Build history of the part. All positions in model axes, mm. A direction names the side the tool comes from. Round coordinates to 2 decimals unless told otherwise and drop trailing zeros. Write each loop counter-clockwise with the first axis right and the second up, starting at its lowest first coordinate (ties: lowest second). Pieces come first, ordered by that corner, then holes. Notation, with made-up numbers: M 50.5,72.25 L 89.5,72.25 A26 cw 89.5,100.25 Z; hole C 31,-17.5 d11. An arc over 180 degrees is marked long. Use a Markdown table: item, result.
from build123d import *

# Parameters (mm, degrees)
SKETCH1_R           = 5
BOSS_EXTRUDE1_DEPTH = 30
CUT_EXTRUDE1_DEPTH  = 1


with BuildPart() as part:
    # Sketch1 → Boss-Extrude1 (new body)
    with BuildSketch(Plane(origin=(0, 0, 0), x_dir=(1, 0, 0), z_dir=(0, 1, 0))):
        Circle(SKETCH1_R)
    extrude(amount=BOSS_EXTRUDE1_DEPTH)

    # Sketch2 → Cut-Extrude1 (cut)
    with BuildSketch(Plane(origin=(0, 30, 0), x_dir=(1, 0, 0), z_dir=(0, 1, 0))):
        Polygon((-1.836629209, 1.610053215), (-1.189493792, 1.610053215), (-1.189493792, -1.889946785), (-1.503596356, -1.889946785), (-1.503596356, 1.251078856), (-2.042057895, 1.251078856), align=None)
        with BuildLine():
            add(Edge.make_bspline(
                [(0.111788259, -0.141349029), (0.112116277, -0.085251641), (0.112753457, 0.023718343), (0.119841878, 0.182502986), (0.131617221, 0.331463275), (0.147754593, 0.470606341), (0.167392574, 0.599968105), (0.19360806, 0.719202862), (0.223420863, 0.828862469), (0.257973309, 0.929304517), (0.296961098, 1.02188222), (0.339395358, 1.108307422), (0.386960153, 1.188449354), (0.436937066, 1.263587144), (0.491349137, 1.332490839), (0.548647928, 1.396133502), (0.611069804, 1.453044252), (0.676492812, 1.504890555), (0.745509277, 1.550340026), (0.816151943, 1.590372765), (0.888907049, 1.624572632), (0.963973232, 1.651463068), (1.04067579, 1.673673915), (1.119282856, 1.688862862), (1.19992422, 1.698419771), (1.254355655, 1.699333439), (1.281960535, 1.699796805)],
                knots=[0, 0, 0, 0, 0.000168282, 0.000326891, 0.000476705, 0.00061646, 0.000747059, 0.00086904, 0.000982494, 0.001087814, 0.001187428, 0.001283689, 0.001376399, 0.001466822, 0.001554203, 0.001639568, 0.001723424, 0.001807301, 0.001889751, 0.001971063, 0.002050735, 0.002130583, 0.002210036, 0.002290062, 0.002370508, 0.002453288, 0.002453288, 0.002453288, 0.002453288], degree=3))
            add(Edge.make_bspline(
                [(1.281960535, 1.699796805), (1.309796013, 1.69930899), (1.365152022, 1.698338879), (1.446992397, 1.689014936), (1.526942079, 1.673543813), (1.604660218, 1.651622839), (1.680785204, 1.624427162), (1.754721612, 1.590340045), (1.826928694, 1.550661177), (1.896258981, 1.5040373), (1.963473596, 1.452055024), (2.026921559, 1.393292355), (2.086608645, 1.328342636), (2.143283951, 1.257900772), (2.195339548, 1.180615687), (2.24491298, 1.097831577), (2.289285016, 1.008100712), (2.332019691, 0.912920245), (2.368906678, 0.809656586), (2.402172923, 0.698891825), (2.429051892, 0.579317638), (2.451441164, 0.451561393), (2.46878606, 0.31515391), (2.481418702, 0.170387594), (2.488091787, 0.017167204), (2.489348488, -0.087590645), (2.489993387, -0.141349029)],
                knots=[0, 0, 0, 0, 8.3481e-05, 0.000166017, 0.000246731, 0.000327534, 0.000408041, 0.000488986, 0.000571522, 0.000654944, 0.000739373, 0.000826202, 0.000914021, 0.001003809, 0.001097153, 0.001193347, 0.001293057, 0.001397277, 0.001506176, 0.001621751, 0.001744038, 0.001873599, 0.002010742, 0.002156422, 0.002309427, 0.002470709, 0.002470709, 0.002470709, 0.002470709], degree=3))
            add(Edge.make_bspline(
                [(2.489993387, -0.141349029), (2.489341803, -0.194872936), (2.488072217, -0.299162088), (2.48149351, -0.451693064), (2.468534879, -0.595691107), (2.452324891, -0.731501569), (2.429873928, -0.858559188), (2.402268761, -0.977303637), (2.371618439, -1.088247708), (2.333783644, -1.19048252), (2.292372934, -1.285434243), (2.247317738, -1.374101391), (2.199047912, -1.457267684), (2.146459167, -1.534267431), (2.090405754, -1.605646088), (2.029687965, -1.670143711), (1.96601738, -1.729314382), (1.898604964, -1.78196601), (1.828193413, -1.828050815), (1.756234336, -1.869264665), (1.681450952, -1.90249736), (1.605538, -1.931032401), (1.527409634, -1.952832853), (1.447163243, -1.967906708), (1.365207007, -1.978478557), (1.309805442, -1.979285037), (1.281960535, -1.979690375)],
                knots=[0, 0, 0, 0, 0.000160581, 0.000312886, 0.000457868, 0.000594226, 0.000723097, 0.000844701, 0.000959884, 0.001068125, 0.001171421, 0.001270505, 0.001366343, 0.001459687, 0.001550023, 0.00163832, 0.001725149, 0.001810562, 0.001894568, 0.001977446, 0.00205903, 0.002139777, 0.00222058, 0.002301983, 0.002384599, 0.00246808, 0.00246808, 0.00246808, 0.00246808], degree=3))
            add(Edge.make_bspline(
                [(1.281960535, -1.979690375), (1.254356421, -1.979224019), (1.199926496, -1.978304457), (1.119274071, -1.968790726), (1.040991627, -1.953495223), (0.964692873, -1.932078618), (0.889986358, -1.905863782), (0.817890071, -1.871710099), (0.747602388, -1.83237603), (0.679310832, -1.787580608), (0.614298671, -1.736258925), (0.552200065, -1.679494636), (0.494575046, -1.615871225), (0.440940951, -1.546393302), (0.389966862, -1.47170006), (0.343077489, -1.390771687), (0.299706635, -1.303929076), (0.260063144, -1.210611165), (0.224914481, -1.109456238), (0.193866773, -0.999307059), (0.169352615, -0.879191423), (0.14836966, -0.750074056), (0.131445277, -0.611400125), (0.119890952, -0.463094347), (0.112749637, -0.305249138), (0.112114566, -0.196979364), (0.111788259, -0.141349029)],
                knots=[0, 0, 0, 0, 8.278e-05, 0.000163226, 0.000243252, 0.00032184, 0.00040079, 0.000480463, 0.00056082, 0.000642298, 0.000725191, 0.000809047, 0.000894412, 0.000982346, 0.001072188, 0.001165503, 0.001262704, 0.001363236, 0.001469448, 0.001583766, 0.001706286, 0.001836995, 0.001976138, 0.002125253, 0.002283161, 0.002450041, 0.002450041, 0.002450041, 0.002450041], degree=3))
        make_face()
        with BuildLine():
            add(Edge.make_bspline(
                [(0.425890823, -0.139946785), (0.42601027, -0.186695484), (0.426242094, -0.277425529), (0.432298294, -0.40926879), (0.440548526, -0.532239118), (0.451189823, -0.646492655), (0.466992772, -0.751642667), (0.48469956, -0.84841235), (0.506247649, -0.936289587), (0.531742667, -1.015877398), (0.560781764, -1.088526467), (0.592487628, -1.156127682), (0.626548351, -1.219479618), (0.664667501, -1.278013227), (0.706182564, -1.331919391), (0.750155824, -1.382152223), (0.798228408, -1.426949204), (0.86473215, -1.480676059), (0.952528625, -1.536195193), (1.06314908, -1.584541283), (1.176817531, -1.614923739), (1.253968781, -1.618787495), (1.292477362, -1.620716016)],
                knots=[0, 0, 0, 0, 0.000140231, 0.000272162, 0.000395845, 0.00050998, 0.000616273, 0.00071473, 0.000805025, 0.000887508, 0.000965234, 0.00103957, 0.001111417, 0.001180842, 0.001248855, 0.001315406, 0.001380877, 0.0014457, 0.001571746, 0.00169106, 0.001806864, 0.001922266, 0.001922266, 0.001922266, 0.001922266], degree=3))
            add(Edge.make_bspline(
                [(1.292477362, -1.620716016), (1.331235033, -1.619118235), (1.408670357, -1.615925972), (1.521804152, -1.585127235), (1.631634422, -1.538657695), (1.717706362, -1.48371019), (1.783188906, -1.43138186), (1.830105896, -1.386767212), (1.873167944, -1.336811345), (1.914010019, -1.282912049), (1.951469095, -1.224039565), (1.985532232, -1.160476989), (2.01661558, -1.092047811), (2.034324626, -1.044278072), (2.043378804, -1.019854638)],
                knots=[0, 0, 0, 0, 0.000116044, 0.000231848, 0.000349318, 0.000472837, 0.000536674, 0.000600645, 0.000666733, 0.000734322, 0.000803367, 0.000875831, 0.000950509, 0.001028633, 0.001028633, 0.001028633, 0.001028633], degree=3))
            add(Edge.make_bspline(
                [(2.043378804, -1.019854638), (2.053930572, -0.988624898), (2.075355186, -0.925215134), (2.10296696, -0.826851482), (2.124712359, -0.723648718), (2.144275725, -0.616223601), (2.157628781, -0.5037839), (2.168376594, -0.386677516), (2.174707281, -0.264816154), (2.175492032, -0.182021163), (2.175890823, -0.139946785)],
                knots=[0, 0, 0, 0, 9.8886e-05, 0.00020078, 0.000306259, 0.000415188, 0.00052824, 0.000645799, 0.000767957, 0.000894177, 0.000894177, 0.000894177, 0.000894177], degree=3))
            add(Edge.make_bspline(
                [(2.175890823, -0.139946785), (2.175340634, -0.097879212), (2.174264346, -0.015586048), (2.170150359, 0.104932133), (2.159526784, 0.219399894), (2.147727665, 0.328310367), (2.130330444, 0.431060669), (2.111572637, 0.528510975), (2.086371425, 0.619453999), (2.05945165, 0.705313581), (2.028641254, 0.785114236), (1.99472552, 0.859228022), (1.958503761, 0.928012747), (1.919161521, 0.991279688), (1.877165838, 1.049312231), (1.831408289, 1.100946826), (1.783703916, 1.147783794), (1.71688673, 1.201246363), (1.62941244, 1.255758058), (1.520566793, 1.305923818), (1.407296149, 1.334732111), (1.330722695, 1.338793798), (1.292477362, 1.340822446)],
                knots=[0, 0, 0, 0, 0.000126219, 0.000246912, 0.000361616, 0.00047102, 0.00057545, 0.000674176, 0.000768567, 0.000858368, 0.000944043, 0.001024988, 0.001102772, 0.001177091, 0.00124833, 0.001317386, 0.001383826, 0.001448649, 0.001573728, 0.001692043, 0.001806995, 0.001921698, 0.001921698, 0.001921698, 0.001921698], degree=3))
            add(Edge.make_bspline(
                [(1.292477362, 1.340822446), (1.25376677, 1.338790999), (1.176275064, 1.334724405), (1.061827109, 1.306031151), (0.952122758, 1.256018186), (0.864879783, 1.201065813), (0.798015996, 1.148727502), (0.750933303, 1.103341048), (0.706787131, 1.053694793), (0.666119431, 0.999292878), (0.628030148, 0.940827511), (0.593049135, 0.877838746), (0.561531805, 0.810007382), (0.532447269, 0.737390947), (0.506874481, 0.657810002), (0.485780518, 0.570041009), (0.466293465, 0.473579117), (0.452498196, 0.367859609), (0.44023444, 0.253577456), (0.432353092, 0.130300137), (0.426221835, -0.001764243), (0.42600337, -0.092963402), (0.425890823, -0.139946785)],
                knots=[0, 0, 0, 0, 0.000116101, 0.000232413, 0.000351368, 0.000476447, 0.000540832, 0.000605795, 0.000672346, 0.000739935, 0.00080936, 0.000881545, 0.00095588, 0.001033607, 0.001116089, 0.001206384, 0.001304286, 0.001411174, 0.001526077, 0.001649061, 0.001781692, 0.001922624, 0.001922624, 0.001922624, 0.001922624], degree=3))
        make_face(mode=Mode.SUBTRACT)
    extrude(amount=-CUT_EXTRUDE1_DEPTH, mode=Mode.SUBTRACT)


solid = part.part
Q1. Cut at B-B on x = -4. Give the cut face in (y, z), and give its area (3 significant figures).
Response values:
| item | result |
|---|---|
| outline | M 0,-3 L 30,-3 L 30,3 L 0,3 Z |
| area | 180 mm2 |
Q2. Cut at C-C on z = -3.25. Give the cut face in (x, y), and give its area (3 significant figures).
Response values:
| item | result |
|---|---|
| outline | M -3.8,0 L 3.8,0 L 3.8,30 L -3.8,30 Z |
| area | 228 mm2 |
Q3. Drop flat-ended pins along their axis: P1, Ø0.8, axis at y = 29.5, z = 1, coming from the +X side; P2, Ø0.5, axis at x = -1.5, y = 29.5, coming from the +Z side; P3, Ø2, axis at y = 6.5, z = -1.5, coming from the -X side. Give the stop position or say it passes through.
Response values:
| item | result |
|---|---|
| P1 | stops at x = 4.96 |
| P2 | stops at z = 4.84 |
| P3 | stops at x = -4.97 |
Q4. Which spindle directions (+Z, -Z, +X, -X, +Y, -Y) get a long thin tool onto all of the face, cutting with end or side? Do faces 1 (the flat face through (-1.504, 29.5, 0.3)), 2 (the flat face through (-0.1, 30, -0.1)). Say none if no direction does.
Response values:
| item | result |
|---|---|
| face 1 | +Y |
| face 2 | +Z, -Z, +X, -X, +Y |
Q5. Cut at A-A on y = 25.5. Give the cut face in (x, z).
Response values:
| item | result |
|---|---|
| outline | C 0,0 d10 |
Q6. Drill centre lines: L1, parallel to Z at x = -0.25, y = 10; L2, parallel to X at y = 14.5, z = -0.5; L3, parallel to X at y = 11.5, z = 1.5. Where is each one in solid material? Low to high.
Response values:
| item | result |
|---|---|
| L1 | z = -4.99 to 4.99 |
| L2 | x = -4.97 to 4.97 |
| L3 | x = -4.77 to 4.77 |
Q7. Two-plate mould, pull along Z, no slides. Class faces 3 (the cylindrical face through (-1.08, 14.79, 4.88)), 4 (the flat face through (1, 30, 0)), 5 (the flat face through (-1.189, 29.5, 0.1)): +Z half, -Z half, draft (parallel to the pull), parting line (faces both ways), or undercut.
Response values:
| item | result |
|---|---|
| face 3 | parting line |
| face 4 | draft |
| face 5 | undercut |
